Build history of the part. All positions in model axes, mm. A direction names the side the tool comes from. Round coordinates to 2 decimals unless told otherwise and drop trailing zeros. Write each loop counter-clockwise with the first axis right and the second up, starting at its lowest first coordinate (ties: lowest second). Pieces come first, ordered by that corner, then holes.
from build123d import *

# Parameters (mm, degrees)
SKETCH1_W           = 3
SKETCH1_H           = 150
SKETCH1_R           = 0.55
SKETCH1_R_2         = 0.25
BOSS_EXTRUDE3_DEPTH = 0.8
SKETCH2_W           = 10
SKETCH2_H           = 3
BOSS_EXTRUDE4_DEPTH = 1


with BuildPart() as part:
    # Sketch1 → Boss-Extrude3 (new body)
    with BuildSketch(Plane.XY):
        with Locations((0, 72.5)):
            Rectangle(SKETCH1_W, SKETCH1_H)
        Circle(SKETCH1_R, mode=Mode.SUBTRACT)
        with Locations((0, 144.5)):
            Circle(SKETCH1_R_2, mode=Mode.SUBTRACT)
        with Locations((0, 134.5)):
            Circle(SKETCH1_R_2, mode=Mode.SUBTRACT)
        with Locations((0, 124.5)):
            Circle(SKETCH1_R_2, mode=Mode.SUBTRACT)
        with Locations((0, 114.5)):
            Circle(SKETCH1_R_2, mode=Mode.SUBTRACT)
        with Locations((0, 104.5)):
            Circle(SKETCH1_R_2, mode=Mode.SUBTRACT)
        with Locations((0, 64.5)):
            Circle(SKETCH1_R_2, mode=Mode.SUBTRACT)
        with Locations((0, 54.5)):
            Circle(SKETCH1_R_2, mode=Mode.SUBTRACT)
        with Locations((0, 94.5)):
            Circle(SKETCH1_R_2, mode=Mode.SUBTRACT)
        with Locations((0, 84.5)):
            Circle(SKETCH1_R_2, mode=Mode.SUBTRACT)
        with Locations((0, 74.5)):
            Circle(SKETCH1_R_2, mode=Mode.SUBTRACT)
        with Locations((0, 44.5)):
            Circle(SKETCH1_R_2, mode=Mode.SUBTRACT)
    extrude(amount=BOSS_EXTRUDE3_DEPTH)

    # Sketch2 → Boss-Extrude4 (add)
    with BuildSketch(Plane.XY.offset(0.8)):
        with Locations((3.5, 4)):
            Rectangle(SKETCH2_W, SKETCH2_H)
    extrude(amount=BOSS_EXTRUDE4_DEPTH)


solid = part.part
1) Wall check: L1, parallel to X at y = 114.5, z = 0.3; L2, parallel to X at y = 108.5, z = 0.3; L3, parallel to Z at x = -0.75, y = 63.5. Give the ranges that are in metal, low to high.
Results:
L1: x = -1.5 to -0.25, 0.25 to 1.5
L2: x = -1.5 to 1.5
L3: z = 0 to 0.8
2) Slice it at B-B (x = 3.75). Write the cut outline in (y, z).
Results:
outline: (2.5, 0.8) - (5.5, 0.8) - (5.5, 1.8) - (2.5, 1.8) - close
3) Slice it at A-A (z = 0.3). Count the separate pieces of the cut face and the enclosed holes in it, plus the area to 3 significant figures.
Results:
separate pieces: 1
enclosed holes: 12
area: 447 mm2
4) Slice it at C-C (y = 10). Write the cut outline in (x, z).
Results:
outline: (-1.5, 0) - (1.5, 0) - (1.5, 0.8) - (-1.5, 0.8) - close
5) Pin check, flat tips, straight feed: pin 1 Ø5 at (x, y) = (2.5, 54) entering from +Z; pin 2 Ø3.5 at (x, y) = (6, 3.5) entering from -Z; pin 3 Ø0.8 at (x, z) = (6, 1.5) entering from -Y. Stop position of each tip, or through.
Results:
pin 1: stops at z = 0.8
pin 2: stops at z = 0.8
pin 3: stops at y = 2.5
6) Which spindle directions (+Z, -Z, +X, -X, +Y, -Y) get a long thin tool onto all of the face, cutting with end or side? Do faces 1 (the flat face through (0, 1, 0.8)), 2 (the flat face through (0, 77, 0.8)), 3 (the flat face through (5, 4, 0.8)). Say none if no direction does.
Results:
face 1: +Z, +X, -X, -Y
face 2: +Z, +X, -X, +Y
face 3: -Z, +X, +Y, -Y
